```python
from build123d import *

# Parameters (mm, degrees)
F0_R      = 9.5
F1_DEPTH  = 16.9
F2_R      = 6
F3_DEPTH  = 1.25
F4_R      = 2
F5_DEPTH  = 12.25
F6_W      = 1.523732
F6_H      = 5.739091
F7_DEPTH  = 8
F8_R      = 3.5
F9_DEPTH  = 2
F10_R     = 1.5
F11_DEPTH = 10


with BuildPart() as f1:
    # F0 (on Front) → F1 (new body)
    with BuildSketch(Plane.XZ):
        Circle(F0_R)
    extrude(amount=F1_DEPTH)

    # F2 (on face) → F3 (join)
    with BuildSketch(Plane.XZ.offset(16.9)):
        Circle(F2_R)
    extrude(amount=F3_DEPTH)

    # F4 (on face) → F5 (join)
    with BuildSketch(Plane.XZ.offset(18.15)):
        Circle(F4_R)
    extrude(amount=F5_DEPTH)

    # F6 (on face) → F7 (cut)
    with BuildSketch(Plane.XZ.offset(30.4)):
        with Locations((-1.998623, 0.154332)):
            Rectangle(F6_W, F6_H)
    extrude(amount=-F7_DEPTH, mode=Mode.SUBTRACT)

    # F8 (on face) → F9 (cut)
    with BuildSketch(Plane(origin=(0, 0, 0), x_dir=(-1, 0, 0), z_dir=(0, 1, 0))):
        Circle(F8_R)
    extrude(amount=-F9_DEPTH, mode=Mode.SUBTRACT)

    # F10 (on face) → F11 (cut)
    with BuildSketch(Plane(origin=(0, -2, 0), x_dir=(-1, 0, 0), z_dir=(0, 1, 0))):
        Circle(F10_R)
    extrude(amount=-F11_DEPTH, mode=Mode.SUBTRACT)


solid = f1.part
```
Check sheet for the modelled part. Datum: model origin and axes. Units: mm. A direction names the side the tool comes from. Round coordinates to 2 decimals unless told otherwise and drop trailing zeros. Loops run counter-clockwise (first coordinate to the right, second up) from the corner with the lowest first, then second, coordinate; pieces in that order, holes last. Notation, with made-up numbers: M 1,74 L 53,74 A24 ccw 53,94 Z; hole C 37,86.25 d6. An arc over 180 degrees is marked long. Answer as a JSON object with one key per item and string values.
1. Access from +Z, -Z, +X, -X, +Y, -Y to the whole of each face (thin tool, end or side, straight path). Record for faces 1 (the cylindrical face through (1.5, -6.93, 0.07)), 2 (the flat face through (-0.1, -16.9, -6.2)), 3 (the flat face through (-1.237, -26, 0)).
Reply:
{"face 1": "+Y", "face 2": "-Y", "face 3": "+Z, -Z, -X, -Y"}
2. Section check B-B (x = 0). Record the boundary of the cut face in (y, z).
Reply:
{"outline": "M -30.4,-2 L -18.15,-2 L -18.15,-6 L -16.9,-6 L -16.9,-9.5 L 0,-9.5 L 0,-3.5 L -2,-3.5 L -2,-1.5 L -12,-1.5 L -12,1.5 L -2,1.5 L -2,3.5 L 0,3.5 L 0,9.5 L -16.9,9.5 L -16.9,6 L -18.15,6 L -18.15,2 L -30.4,2 Z"}
3. Scan lines: line 1 (Z direction, x = 0, y = -1); line 2 (Z direction, x = 0, y = -5.5); line 3 (Y direction, x = 3, z = 1). Record each from-to range of solid material in increasing order.
Reply:
{"line 1": "z = -9.5 to -3.5, 3.5 to 9.5", "line 2": "z = -9.5 to -1.5, 1.5 to 9.5", "line 3": "y = -18.15 to -2"}
4. Section check D-D (y = -16). Record the boundary of the cut face in (x, z).
Reply:
{"outline": "C 0,0 d19"}
5. Section check C-C (y = -5.5). Record the boundary of the cut face in (x, z), plus the area to 3 significant figures.
Reply:
{"outline": "C 0,0 d19; hole C 0,0 d3", "area": "276 mm²"}
6. Mould release check, pull along Z, two halves, no side actions. Record for faces 4 (the cylindrical face through (-5.994, -17.516, 0.264)), 5 (the flat face through (0, -12, 0)), 6 (the flat face through (0, -30.4, 0)): pulls with the +Z half, pulls with the -Z half, needs draft (parallel to the pull), parting line crosses it, or undercut.
Reply:
{"face 4": "parting line crosses it", "face 5": "undercut", "face 6": "needs draft"}
7. Section check A-A (z = 0). Record the boundary of the cut face in (x, y), plus the area to 3 significant figures.
Reply:
{"outline": "M -9.5,-16.9 L -6,-16.9 L -6,-18.15 L -2,-18.15 L -2,-22.4 L -1.24,-22.4 L -1.24,-30.4 L 2,-30.4 L 2,-18.15 L 6,-18.15 L 6,-16.9 L 9.5,-16.9 L 9.5,0 L 3.5,0 L 3.5,-2 L 1.5,-2 L 1.5,-12 L -1.5,-12 L -1.5,-2 L -3.5,-2 L -3.5,0 L -9.5,0 Z", "area": "335 mm²"}
8. Gauge pin test, flat ends, axial feed: P1, Ø3, axis at y = -22.5, z = 3, coming from the +X side; P2, Ø1.5, axis at x = -0.5, z = -0.5, coming from the +Y side; P3, Ø5, axis at y = -23.5, z = -0.5, coming from the +X side. Record the tip position at first contact, or that the pin passes through.
Reply:
{"P1": "stops at x = 1.32", "P2": "stops at y = -12", "P3": "stops at x = 2"}
